Part model, mm, in its own coordinate system. Face numbers are marked on the shaded views. A direction names the side the tool comes from. Round coordinates to 2 decimals unless told otherwise and drop trailing zeros. Loops run counter-clockwise (first coordinate to the right, second up) from the corner with the lowest first, then second, coordinate; pieces in that order, holes last. Notation, with made-up numbers: M 57.25,56.5 L 74.25,56.5 A32 cw 74.25,95.5 Z; hole C -38,-24 d5. An arc over 180 degrees is marked long. Write each question's results on one line, items separated by ' | '.
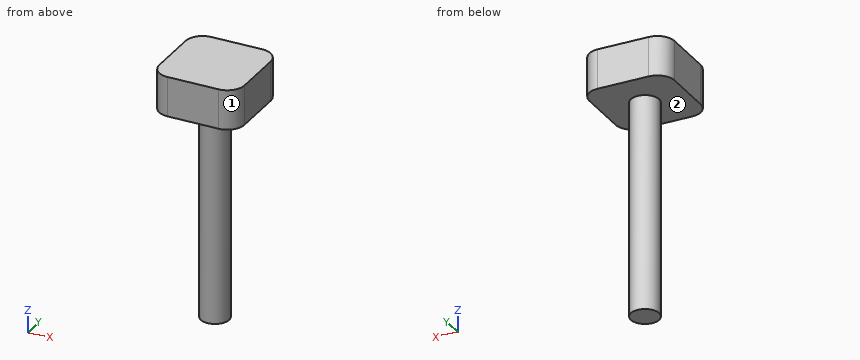
from build123d import *

# Parameters (mm, degrees)
SKETCH138_R  = 2.5
PAD069_DEPTH = 45
SKETCH139_W  = 15
SKETCH139_H  = 15
PAD070_DEPTH = 7
FILLET_R     = 3


with BuildPart() as part:
    # Sketch138 → Pad069 (new body)
    with BuildSketch(Plane.XY):
        Circle(SKETCH138_R)
    extrude(amount=PAD069_DEPTH)

    # Sketch139 (on Face3 of Pad069) → Pad070 (join)
    with BuildSketch(Plane.XY.offset(45)):
        Rectangle(SKETCH139_W, SKETCH139_H)
    extrude(amount=-PAD070_DEPTH)

    # Fillet
    fillet_edges = [part.edges().sort_by_distance(p)[0] for p in [
        (7.5, -7.5, 41.5),
        (7.5, 7.5, 41.5),
        (-7.5, 7.5, 41.5),
        (-7.5, -7.5, 41.5),
    ]]
    fillet(fillet_edges, radius=FILLET_R)


with BuildPart() as part_1:
    # Body040 placement: moved
    add(part.part.moved(Location((0, 0, 20))))


solid = part_1.part
Item 1: Wall check: L1, parallel to Z at x = -6.5, y = 1; L2, parallel to X at y = 1.75, z = 41.5; L3, parallel to Y at x = -0.75, z = 32. Give the ranges that are in metal, low to high.
Filled sheet:
L1: 58 to 65 | L2: -1.79 to 1.79 | L3: -2.38 to 2.38
Item 2: Band-saw the part on D-D on x = 3. Give the cut face in (y, z).
Filled sheet:
outline: M -7.5,58 L 7.5,58 L 7.5,65 L -7.5,65 Z
Item 3: Band-saw the part on A-A on y = 0. Give the cut face in (x, z), and give its area (3 significant figures).
Filled sheet:
outline: M -7.5,58 L -2.5,58 L -2.5,20 L 2.5,20 L 2.5,58 L 7.5,58 L 7.5,65 L -7.5,65 Z | area: 295 mm^2
Item 4: Which spindle directions (+Z, -Z, +X, -X, +Y, -Y) get a long thin tool onto all of the face, cutting with end or side? Do the marked faces 1 and 2. Say none if no direction does.
Filled sheet:
face 1: +Z, -Z, +X, -Y | face 2: -Z
Item 5: Band-saw the part on C-C on z = 50.5. Give the cut face in (x, y), and give its area (3 significant figures).
Filled sheet:
outline: C 0,0 d5 | area: 19.6 mm^2
Item 6: Drop flat-ended pins along their axis: P1, Ø2, axis at x = 1.5, z = 38.5, coming from the -Y side; P2, Ø3, axis at y = -1, z = 45.5, coming from the -X side; P3, Ø4, axis at y = -4, z = 29, coming from the -X side. Give the stop position or say it passes through.
Filled sheet:
P1: y = -2.45 | P2: x = -2.5 | P3: x = -1.5
